Check sheet for the drawn part. Datum: minimum x, y, z corner. Units: mm. A direction names the side the tool comes from. Round coordinates to 2 decimals unless told otherwise and drop trailing zeros. Loops run counter-clockwise (first coordinate to the right, second up) from the corner with the lowest first, then second, coordinate; pieces in that order, holes last. Notation, with made-up numbers: (12, -33) -> (59, -33) arc R16 ccw to (59, -14) -> close; hole circle Ø8 at (71, 7). An arc over 180 degrees is marked (long way). Return JSON: item names as keys, results as strings.
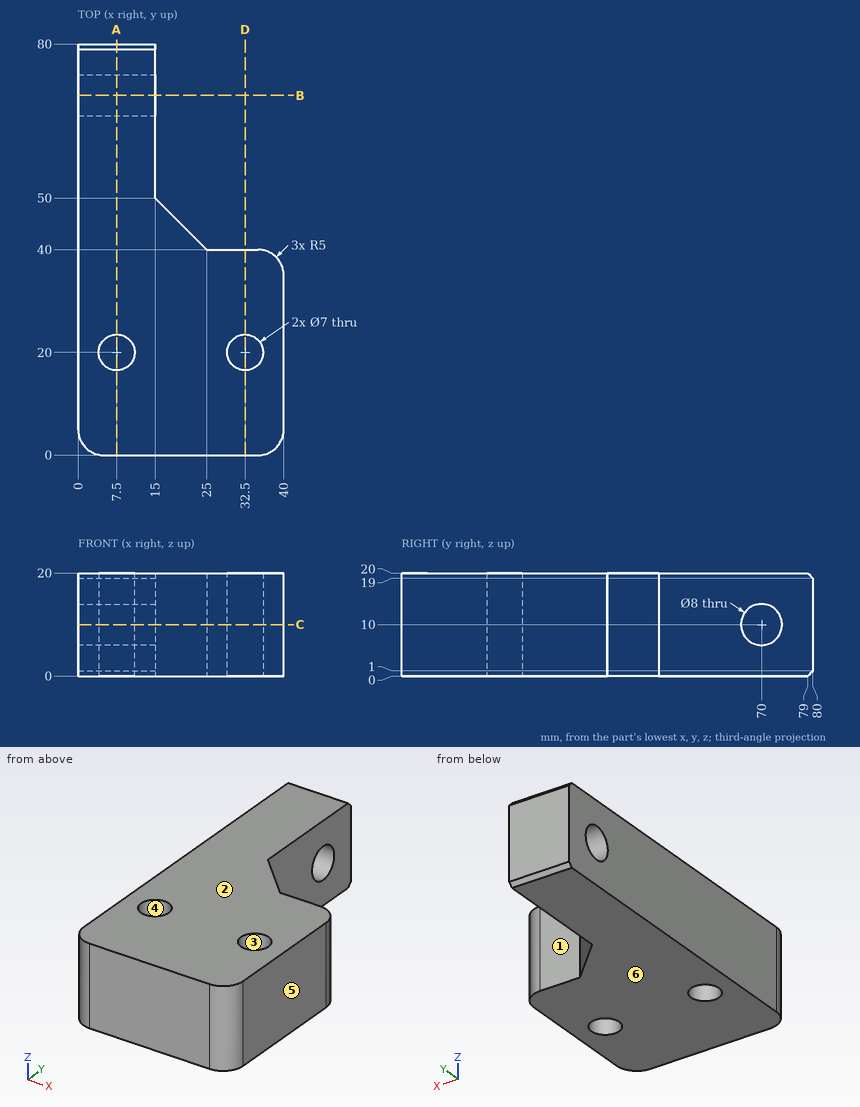
Q1. Draft check along X on the marked faces 3, 4, 5 and 6. Enter one of: released by +X, released by -X, zero draft, split by the parting line, or undercut.
Results list:
{"face 3": "undercut", "face 4": "undercut", "face 5": "released by +X", "face 6": "zero draft"}
Q2. Section check D-D (x = 32.5). Record the boundary of the cut face in (y, z).
Results list:
{"outline": "(0, 0) -> (16.5, 0) -> (16.5, 20) -> (0, 20) -> close; (23.5, 0) -> (40, 0) -> (40, 20) -> (23.5, 20) -> close"}
Q3. Section check B-B (y = 70). Record the boundary of the cut face in (x, z), then the cut area to 3 significant figures.
Results list:
{"outline": "(0, 0) -> (15, 0) -> (15, 6) -> (0, 6) -> close; (0, 14) -> (15, 14) -> (15, 20) -> (0, 20) -> close", "area": "180 mm^2"}
Q4. Tool access check on the marked faces 1 and 2. Record the directions out of +Z, -Z, +X, -X, +Y, -Y that give a thin tool (end or side, any length) a straight path to the whole face; none if there is none.
Results list:
{"face 1": "+Z, -Z, +X, +Y", "face 2": "+Z, +X, -X, +Y, -Y"}
Q5. Section check C-C (z = 10). Record the boundary of the cut face in (x, y).
Results list:
{"outline": "(0, 5) arc R5 ccw to (5, 0) -> (35, 0) arc R5 ccw to (40, 5) -> (40, 35) arc R5 ccw to (35, 40) -> (25, 40) -> (15, 50) -> (15, 66) -> (0, 66) -> close; (0, 74) -> (15, 74) -> (15, 80) -> (0, 80) -> close; hole circle Ø7 at (7.5, 20); hole circle Ø7 at (32.5, 20)"}
Q6. Material ranges on line 1 (Y direction, x = 32.5, z = 14.5); line 2 (Y direction, x = 6, z = 11.75); line 3 (Y direction, x = 7.5, z = 7.25), recorded low to high.
Results list:
{"line 1": "0 to 16.5, 23.5 to 40", "line 2": "0 to 16.84, 23.16 to 66.4, 73.6 to 80", "line 3": "0 to 16.5, 23.5 to 67.1, 72.9 to 80"}
Q7. Go/stop test with flat-tipped pins: pin 1 (8 mm diameter, centred on y = 59.5, z = 4.5, fed in from +X); pin 2 (8 mm diameter, centred on x = 31.5, z = 12, fed in from +Y); pin 3 (7 mm diameter, centred on y = 70, z = 10, fed in from -X); pin 4 (12 mm diameter, centred on y = 44.5, z = 2, fed in from +X). Record where each tip stops, or that it passes through.
Results list:
{"pin 1": "x = 15", "pin 2": "y = 40", "pin 3": "through", "pin 4": "x = 38.57"}
Q8. Section check A-A (x = 7.5). Record the boundary of the cut face in (y, z).
Results list:
{"outline": "(0, 0) -> (16.5, 0) -> (16.5, 20) -> (0, 20) -> close; (23.5, 0) -> (79, 0) -> (80, 1) -> (80, 19) -> (79, 20) -> (23.5, 20) -> close; hole circle Ø8 at (70, 10)"}
